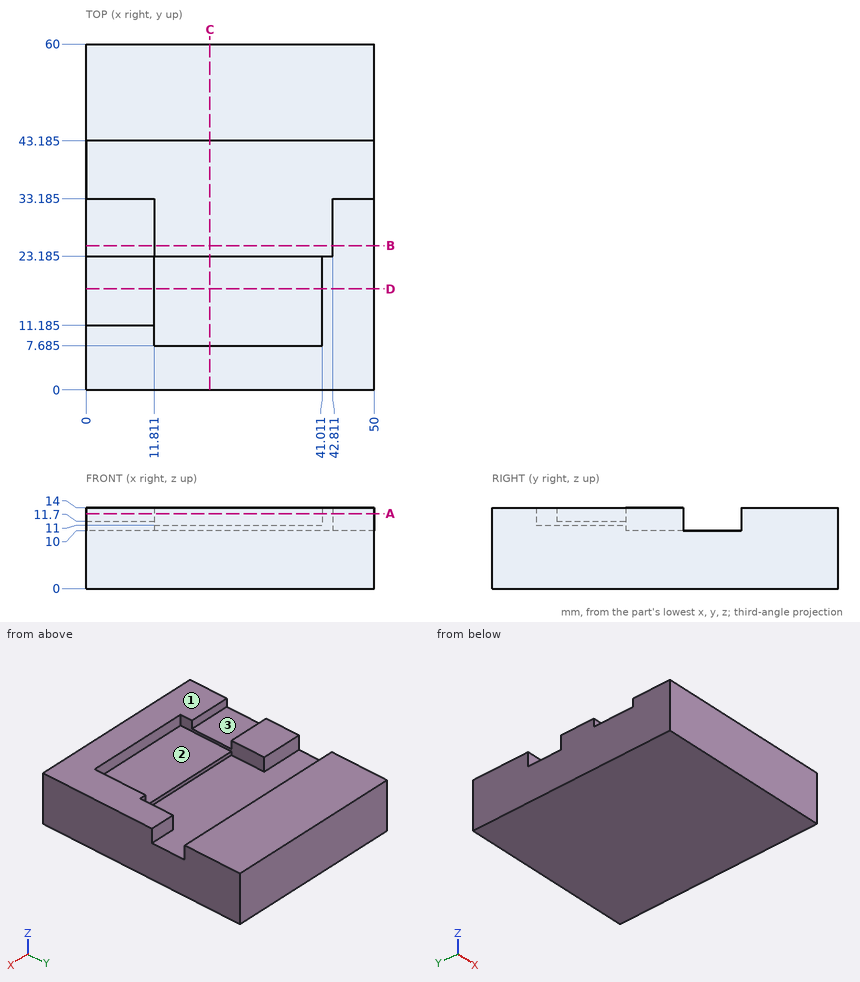
Can you work these out from the drawing? Everything is in mm from the part's minimum corner. A direction names the side the tool comes from. Give positions to 0.01 mm unless a question says otherwise; leave off trailing zeros. Order: outer loops, then holes, each group sorted by start corner. A loop starts at its lowest first (then second) coordinate and runs counter-clockwise, first axis right, second up. Notation, with made-up numbers: M 35.5,-29 L 89.5,-29 A27 cw 89.5,-2 Z; hole C 70,-28.5 d3. An arc over 180 degrees is marked long. Use a Markdown table: item, result. Add a question column.
1. Suppose I cut it at C-C (x = 21.5). List the corners of the cut face in (y, z) for me (1 decimal).
2. Suppose I cut it at B-B (y = 25). List the corners of the cut face in (x, z) for me, and give its area (3 significant figures).
3. Suppose I cut it at D-D (y = 17.5). List the corners of the cut face in (x, z) for me, and give its area (3 significant figures).
4. For pin 1 Ø0.9 at (y, z) = (14, 13) entering from -X; pin 2 Ø12.5 at (x, y) = (28.5, 16.5) entering from +Z, each with a flat end and sliding along its axis, tell me the tip position at first contact or that it passes through.
5. I need wall thicknesses on probe 1 along Y at (x, z) = (46.5, 13.25) (1 decimal); probe 2 along Y at (x, z) = (17.5, 11.5) (1 decimal); probe 3 along Z at (x, y) = (19.5, 35.5). Which ranges of each line are inside material? Lowest first, please. Write a range as from..to.
6. On a 3-axis mill with a long thin cutter (end or side, diameter ignored), from which of +Z, -Z, +X, -X, +Y, -Y can I reach the whole of each face in a straight line? I mean the marked faces 1, 2 and 3. Say none if no direction works.
7. Suppose I cut it at A-A (z = 13). List the corners of the cut face in (x, y) for me (1 decimal), and give its area (3 significant figures).
Results list:
| question | item | result |
|---|---|---|
| 1 | outline | M 0,0 L 60,0 L 60,14 L 43.2,14 L 43.2,10 L 23.2,10 L 23.2,11 L 7.7,11 L 7.7,14 L 0,14 Z |
| 2 | outline | M 0,0 L 50,0 L 50,14 L 42.81,14 L 42.81,10 L 11.81,10 L 11.81,14 L 0,14 Z |
| 2 | area | 576 mm² |
| 3 | outline | M 0,0 L 50,0 L 50,14 L 41.01,14 L 41.01,11 L 11.81,11 L 11.81,11.7 L 0,11.7 Z |
| 3 | area | 585 mm² |
| 4 | pin 1 | stops at x = 41.01 |
| 4 | pin 2 | stops at z = 11 |
| 5 | probe 1 | y = 0..33.2, 43.2..60 |
| 5 | probe 2 | y = 0..7.7, 43.2..60 |
| 5 | probe 3 | z = 0..10 |
| 6 | face 1 | +Z, +X, -X, +Y, -Y |
| 6 | face 2 | +Z |
| 6 | face 3 | +Z, -X |
| 7 | outline | M 0,0 L 50,0 L 50,33.2 L 42.8,33.2 L 42.8,23.2 L 41,23.2 L 41,7.7 L 11.8,7.7 L 11.8,11.2 L 0,11.2 Z; M 0,23.2 L 11.8,23.2 L 11.8,33.2 L 0,33.2 Z; M 0,43.2 L 50,43.2 L 50,60 L 0,60 Z |
| 7 | area | 1,600 mm² |
